Geometry: final body of the model. Coordinates: model frame, mm. Give positions to 0.01 mm unless a question says otherwise; leave off trailing zeros. Write each loop counter-clockwise with the first axis right and the second up, starting at its lowest first coordinate (ties: lowest second). Pieces come first, ordered by that corner, then holes. Notation, with made-up numbers: M -38,65 L 13,65 A19 cw 13,70 Z; hole C -35.75,-25 d11. An arc over 180 degrees is marked long. Use one line per item in the form item = value. Start each with the question number.
Item 1: Section query A-A on x = 0. Return loops of the section in (y, z).
Item 2: Section query C-C on z = 8.25. Return loops of the section in (x, y).
Item 3: Pull-direction query (X, two-part tool) for faces 1 (the flat face through (0, -2.2, 12.5)), 2 (the cylindrical face through (-0.867, -3.905, -0.167)), 3 (the cylindrical face through (0, -2, 0)); classes: released by +X, released by -X, zero draft, split by the parting line, or undercut.
Item 4: Material intervals for line 1 along Y through (x, z) = (0, -6); line 2 along X through (y, z) = (1, -9); line 3 along X through (y, z) = (-0.5, -5.5), sorted ascending. Write a range as from..to.
Item 5: Contact query for a flat-ended pin moving along its axis: P1, Ø3.5, axis at x = 0, y = 0, coming from the -Z side. Output: stop coordinate, or through.
from build123d import *

# Parameters (mm, degrees)
BOSS_EXTRUDE1_DEPTH      = 12.5
BOSS_EXTRUDE1_DEPTH_BACK = 12.5
SKETCH3_R                = 4
CHAMFER1_SIZE            = 0.6
SKETCH4_R                = 2
CUT_EXTRUDE1_DEPTH       = 42


with BuildPart() as part:
    # Sketch3 → Boss-Extrude1 (new, two sides: drawn at the far end of the back side and taken through both)
    with BuildSketch(Plane.XY.offset(-BOSS_EXTRUDE1_DEPTH_BACK)):
        Circle(SKETCH3_R)
    extrude(amount=BOSS_EXTRUDE1_DEPTH + BOSS_EXTRUDE1_DEPTH_BACK)

    # Chamfer1
    chamfer1_edges = [part.edges().sort_by_distance(p)[0] for p in [
        (-4, 0, -12.5),
        (-4, 0, 12.5),
    ]]
    chamfer(chamfer1_edges, length=CHAMFER1_SIZE)

    # Sketch4 → Cut-Extrude1 (cut)
    with BuildSketch(Plane(origin=(0, 0, -12.5), x_dir=(-1, 0, 0), z_dir=(0, 0, -1))):
        Circle(SKETCH4_R)
    extrude(amount=-CUT_EXTRUDE1_DEPTH, mode=Mode.SUBTRACT)


solid = part.part
Answer sheet:
q1.outline = M -4,-11.9 L -3.4,-12.5 L -2,-12.5 L -2,12.5 L -3.4,12.5 L -4,11.9 Z; M 2,-12.5 L 3.4,-12.5 L 4,-11.9 L 4,11.9 L 3.4,12.5 L 2,12.5 Z
q2.outline = C 0,0 d8; hole C 0,0 d4
q3.face_1 = zero draft
q3.face_2 = split by the parting line
q3.face_3 = undercut
q4.line_1 = -4..-2, 2..4
q4.line_2 = -3.87..-1.73, 1.73..3.87
q4.line_3 = -3.97..-1.94, 1.94..3.97
q5.P1 = through
